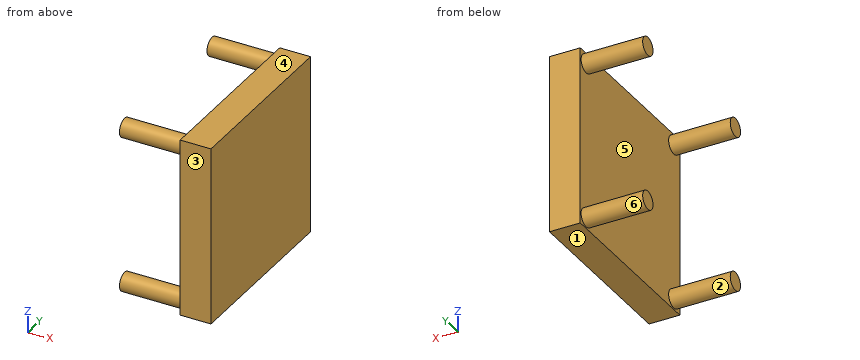
from build123d import *

# Parameters (mm, degrees)
SKETCH1_W           = 29
SKETCH1_H           = 29
BOSS_EXTRUDE1_DEPTH = 5
SKETCH2_R           = 1.5
BOSS_EXTRUDE2_DEPTH = 10


with BuildPart() as part:
    # Sketch1 → Boss-Extrude1 (new body)
    with BuildSketch(Plane(origin=(0, 0, 0), x_dir=(0, 0, -1), z_dir=(1, 0, 0))):
        Rectangle(SKETCH1_W, SKETCH1_H)
    extrude(amount=BOSS_EXTRUDE1_DEPTH)

    # Sketch2 → Boss-Extrude2 (add)
    with BuildSketch(Plane.ZY):
        with Locations((-12.75, 12.75)):
            Circle(SKETCH2_R)
        with Locations((12.75, 12.75)):
            Circle(SKETCH2_R)
        with Locations((12.75, -12.75)):
            Circle(SKETCH2_R)
        with Locations((-12.75, -12.75)):
            Circle(SKETCH2_R)
    extrude(amount=BOSS_EXTRUDE2_DEPTH)


solid = part.part
The model under review builds one solid part; all positions refer to its coordinate system, in mm. Face numbers are marked on the shaded views. A direction names the side the tool comes from. Round coordinates to 2 decimals unless told otherwise and drop trailing zeros. Loops run counter-clockwise (first coordinate to the right, second up) from the corner with the lowest first, then second, coordinate; pieces in that order, holes last. Notation, with made-up numbers: (1, 38.25) -> (20, 38.25) arc R27 ccw to (20, 70.25) -> close; hole circle Ø11 at (46, 47). An arc over 180 degrees is marked (long way). One line per question, with ' | ' between items. Start each with the question number.
Item 1: Add section A-A, the plane z = -12.75. Write out the cut boundary in (x, y), then the cut area to 3 significant figures.
Item 2: Wall thickness on line 1 along X through (y, z) = (-7.5, -4.5); line 2 along Z through (x, y) = (-1.75, -11.5); line 3 along Y through (x, z) = (-2, -12.25): over which ranges is each line inside the solid? List them lowest first. Write a range as [from, to].
Item 3: Draft analysis for pull direction Y (two halves, no side actions). For the marked faces 3, 4, 5 and 6, state which applies: +Y half, -Y half, draft (parallel to the pull), parting line (faces both ways), or undercut.
Item 4: Add section B-B, the plane x = -4.5. Write out the cut boundary in (y, z), then the cut area to 3 significant figures.
Item 5: Machinability: for the marked faces 1 and 2, which of the approach directions +Z, -Z, +X, -X, +Y, -Y give a long, thin tool a straight path to every point of the face, cutting with its end or side? Answer none if there is none.
Item 6: Add section D-D, the plane y = 0. Write out the cut boundary in (x, z).
Return value:
1) outline: (-10, -14.25) -> (0, -14.25) -> (0, -14.5) -> (5, -14.5) -> (5, 14.5) -> (0, 14.5) -> (0, 14.25) -> (-10, 14.25) -> (-10, 11.25) -> (0, 11.25) -> (0, -11.25) -> (-10, -11.25) -> close | area: 205 mm2
2) line 1: x = [0, 5] | line 2: z = [-13.58, -11.92], [11.92, 13.58] | line 3: y = [-14.16, -11.34], [11.34, 14.16]
3) face 3: -Y half | face 4: draft | face 5: undercut | face 6: undercut
4) outline: circle Ø3 at (-12.75, -12.75); circle Ø3 at (-12.75, 12.75); circle Ø3 at (12.75, -12.75); circle Ø3 at (12.75, 12.75) | area: 28.3 mm2
5) face 1: -Z, +X, -X, +Y, -Y | face 2: -X
6) outline: (0, -14.5) -> (5, -14.5) -> (5, 14.5) -> (0, 14.5) -> close
